Work out the finished part from the listing and answer in its coordinate system (mm). Coordinates: 2 decimals unless noted, no trailing zeros. Order: outer loops, then holes, each group sorted by start corner. A loop starts at its lowest first (then second) coordinate and runs counter-clockwise, first axis right, second up. Notation, with made-up numbers: (-31, 8) -> (-20, 8) arc R27 cw to (-20, 39) -> close; hole circle Ø3 at (-3, -37.5). An arc over 180 degrees is marked (long way). Use one line per item in the form item = value.
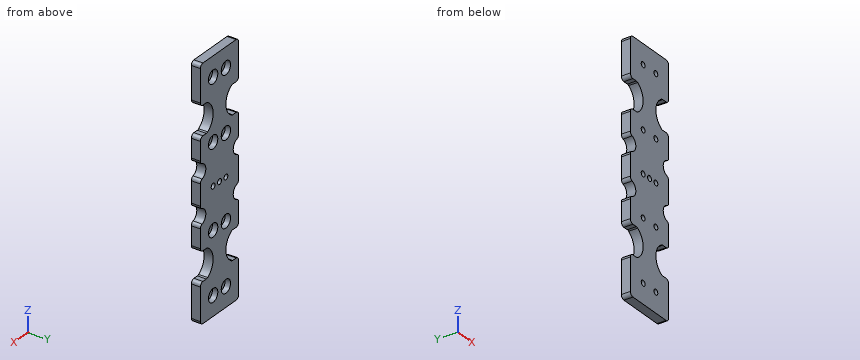
Autodesk Inventor part; units mm, degrees
ref_plane "YZ Plane" through (0, 0, 0) normal (1, 0, 0) x (0, 1, 0)
ref_plane "XZ Plane" through (0, 0, 0) normal (0, 1, 0) x (-1, 0, 0)
ref_plane "XY Plane" through (0, 0, 0) normal (0, 0, 1) x (1, 0, 0)
sketch "Sketch1" plane through (0, 0, 0) normal (0, 1, 0) x (-1, 0, 0)
  line L0 (13.7897, -1.2319) -> (-9.6368, -1.2319) construction
  line L1 (0.7897, 10.3965) -> (0.7897, -17.2319) construction
  line L2 (0.7897, -1.2319) -> (15.7897, -1.2319)
  line L3 (15.7897, -1.2319) -> (15.7897, -7.0606)
  line L4 (15.7897, -8.7319) -> (0.7897, -8.7319)
  line L5 (0.7897, -8.7319) -> (0.7897, -1.2319)
  line L6 (21.7897, -1.2319) -> (-22.2103, -1.2319) construction
  line L7 (0.7897, 17.7681) -> (0.7897, -29.2319) construction
  circle A0 centre (5.7897, -24.2319) radius 3.65
  circle A1 centre (5.7897, -24.2319) radius 5
  circle A2 centre (5.7897, -58.2319) radius 3.65
  circle A3 centre (5.7897, -58.2319) radius 5
  line L8 (0.7897, -17.2319) -> (15.7897, -17.2319)
  line L9 (15.7897, -18.9033) -> (15.7897, -29.2319)
  line L10 (13.7897, -31.2319) -> (11.138, -31.2319)
  line L11 (0.7897, -31.2319) -> (0.7897, -17.2319)
  line L12 (0.7897, -51.2319) -> (15.7897, -51.2319)
  line L13 (15.7897, -51.2319) -> (15.7897, -65.2319)
  line L14 (15.7897, -65.2319) -> (0.7897, -65.2319)
  line L15 (0.7897, -65.2319) -> (0.7897, -51.2319)
  arc A4 (14.4297, -8.9554) -> (14.4297, -17.0085) centre (15.7897, -12.9819) ccw
  line L16 (15.7897, -51.2319) -> (0.7897, -51.2319)
  line L17 (0.7897, -51.2319) -> (0.7897, -47.2319)
  line L18 (11.138, -47.2319) -> (13.7897, -47.2319)
  line L19 (15.7897, -49.2319) -> (15.7897, -51.2319)
  line L20 (15.7897, -65.2319) -> (0.7897, -65.2319)
  line L21 (0.7897, -65.2319) -> (0.7897, -69.2319)
  line L22 (0.7897, -69.2319) -> (13.7897, -69.2319)
  line L23 (15.7897, -67.2319) -> (15.7897, -65.2319)
  arc A5 (14.4297, -8.9554) -> (15.7897, -7.0606) centre (13.7897, -7.0606) ccw
  arc A6 (15.7897, -18.9033) -> (14.4297, -17.0085) centre (13.7897, -18.9033) ccw
  arc A7 (-12.8503, -17.0085) -> (-14.2103, -18.9033) centre (-12.2103, -18.9033) ccw
  circle A8 centre (-4.2103, -24.2319) radius 3.65
  circle A9 centre (-4.2103, -24.2319) radius 5
  line L24 (0.7897, -17.2319) -> (-14.2103, -17.2319)
  arc A10 (-12.8503, -17.0085) -> (-12.8503, -8.9554) centre (-14.2103, -12.9819) ccw
  arc A11 (-14.2103, -7.0606) -> (-12.8503, -8.9554) centre (-12.2103, -7.0606) ccw
  line L25 (-14.2103, -8.7319) -> (0.7897, -8.7319)
  line L26 (-14.2103, -1.2319) -> (-14.2103, -7.0606)
  line L27 (-14.2103, -18.9033) -> (-14.2103, -29.2319)
  line L28 (-12.2103, -31.2319) -> (-9.5586, -31.2319)
  line L29 (-14.2103, -49.2319) -> (-14.2103, -51.2319)
  line L30 (-9.5586, -47.2319) -> (-12.2103, -47.2319)
  line L31 (0.7897, -51.2319) -> (-14.2103, -51.2319)
  line L32 (-14.2103, -51.2319) -> (0.7897, -51.2319)
  line L33 (-14.2103, -51.2319) -> (-14.2103, -65.2319)
  circle A12 centre (-4.2103, -58.2319) radius 3.65
  circle A13 centre (-4.2103, -58.2319) radius 5
  line L34 (-14.2103, -67.2319) -> (-14.2103, -65.2319)
  line L35 (-14.2103, -65.2319) -> (0.7897, -65.2319)
  line L36 (-14.2103, -65.2319) -> (0.7897, -65.2319)
  line L37 (0.7897, -69.2319) -> (-12.2103, -69.2319)
  line L38 (0.7897, 6.2681) -> (0.7897, -1.2319)
  arc A14 (-12.8503, 6.4915) -> (-12.8503, 14.5446) centre (-14.2103, 10.5181) ccw
  line L39 (-14.2103, 6.2681) -> (0.7897, 6.2681)
  line L40 (-14.2103, -1.2319) -> (-14.2103, 4.5967)
  arc A15 (-12.8503, 6.4915) -> (-14.2103, 4.5967) centre (-12.2103, 4.5967) ccw
  line L41 (15.7897, -1.2319) -> (15.7897, 4.5967)
  line L42 (15.7897, 6.2681) -> (0.7897, 6.2681)
  line L43 (0.7897, -12.8604) -> (0.7897, 14.7681) construction
  line L44 (0.7897, -20.2319) -> (0.7897, 26.7681) construction
  circle A16 centre (5.7897, 55.7681) radius 3.65
  circle A17 centre (5.7897, 55.7681) radius 5
  line L45 (0.7897, 48.7681) -> (15.7897, 48.7681)
  line L46 (15.7897, 48.7681) -> (15.7897, 62.7681)
  line L47 (15.7897, 62.7681) -> (0.7897, 62.7681)
  line L48 (0.7897, 62.7681) -> (0.7897, 48.7681)
  line L49 (15.7897, 48.7681) -> (0.7897, 48.7681)
  line L50 (11.138, 44.7681) -> (13.7897, 44.7681)
  line L51 (15.7897, 45.7681) -> (15.7897, 48.7681)
  line L52 (15.7897, 62.7681) -> (0.7897, 62.7681)
  line L53 (0.7897, 66.7681) -> (13.7897, 66.7681)
  line L54 (15.7897, 64.7681) -> (15.7897, 62.7681)
  line L55 (0.7897, 62.7681) -> (0.7897, 66.7681)
  line L56 (13.7897, 28.7681) -> (11.138, 28.7681)
  circle A18 centre (5.7897, 21.7681) radius 3.65
  circle A19 centre (5.7897, 21.7681) radius 5
  line L57 (0.7897, 14.7681) -> (15.7897, 14.7681)
  line L58 (15.7897, 16.4394) -> (15.7897, 27.7681)
  arc A20 (14.4297, 14.5446) -> (14.4297, 6.4915) centre (15.7897, 10.5181) ccw
  arc A21 (15.7897, 4.5967) -> (14.4297, 6.4915) centre (13.7897, 4.5967) ccw
  arc A22 (14.4297, 14.5446) -> (15.7897, 16.4394) centre (13.7897, 16.4394) ccw
  line L59 (0.7897, 14.7681) -> (-14.2103, 14.7681)
  arc A23 (-14.2103, 16.4394) -> (-12.8503, 14.5446) centre (-12.2103, 16.4394) ccw
  circle A24 centre (-4.2103, 21.7681) radius 3.65
  line L60 (-14.2103, 16.4394) -> (-14.2103, 26.7681)
  line L61 (-12.2103, 28.7681) -> (-9.5586, 28.7681)
  line L62 (0.7897, 28.7681) -> (0.7897, 14.7681)
  circle A25 centre (-4.2103, 21.7681) radius 5
  line L63 (0.7897, 66.7681) -> (-12.2103, 66.7681)
  line L64 (-14.2103, 64.7681) -> (-14.2103, 62.7681)
  line L65 (0.7897, 48.7681) -> (0.7897, 44.7681)
  circle A26 centre (-4.2103, 55.7681) radius 3.65
  line L66 (-14.2103, 62.7681) -> (0.7897, 62.7681)
  line L67 (-14.2103, 62.7681) -> (0.7897, 62.7681)
  line L68 (-14.2103, 48.7681) -> (-14.2103, 62.7681)
  line L69 (0.7897, 48.7681) -> (-14.2103, 48.7681)
  line L70 (-14.2103, 48.7681) -> (0.7897, 48.7681)
  line L71 (-14.2103, 46.7681) -> (-14.2103, 48.7681)
  line L72 (-9.5586, 44.7681) -> (-12.2103, 44.7681)
  circle A27 centre (-4.2103, 55.7681) radius 5
  arc A28 (15.7897, 64.7681) -> (13.7897, 66.7681) centre (13.7897, 64.7681) ccw
  arc A29 (-12.2103, 66.7681) -> (-14.2103, 64.7681) centre (-12.2103, 64.7681) ccw
  arc A30 (13.7897, -69.2319) -> (15.7897, -67.2319) centre (13.7897, -67.2319) ccw
  arc A31 (-14.2103, -67.2319) -> (-12.2103, -69.2319) centre (-12.2103, -67.2319) ccw
  arc A32 (10.0879, 44.4702) -> (10.0879, 29.0659) centre (14.8397, 36.7681) ccw
  line L73 (15.7897, 46.7681) -> (15.7897, 45.7681)
  line L74 (15.7897, 26.7681) -> (15.7897, 27.7681)
  arc A33 (13.7897, 44.7681) -> (15.7897, 46.7681) centre (13.7897, 46.7681) ccw
  arc A34 (11.138, 44.7681) -> (10.0879, 44.4702) centre (11.138, 42.7681) ccw
  arc A35 (10.0879, 29.0659) -> (11.138, 28.7681) centre (11.138, 30.7681) ccw
  arc A36 (15.7897, 26.7681) -> (13.7897, 28.7681) centre (13.7897, 26.7681) ccw
  arc A37 (-8.5085, 29.0659) -> (-8.5085, 44.4702) centre (-13.2603, 36.7681) ccw
  line L75 (-14.2103, 45.7681) -> (-14.2103, 44.7681)
  line L76 (-14.2103, 27.7681) -> (-14.2103, 28.7681)
  arc A38 (-8.5085, 44.4702) -> (-9.5586, 44.7681) centre (-9.5586, 42.7681) ccw
  arc A39 (-9.5586, 28.7681) -> (-8.5085, 29.0659) centre (-9.5586, 30.7681) ccw
  arc A40 (-12.2103, 28.7681) -> (-14.2103, 26.7681) centre (-12.2103, 26.7681) ccw
  arc A41 (-14.2103, 46.7681) -> (-12.2103, 44.7681) centre (-12.2103, 46.7681) ccw
  arc A42 (10.0879, -31.5298) -> (10.0879, -46.9341) centre (14.8397, -39.2319) ccw
  arc A43 (-8.5085, -46.9341) -> (-8.5085, -31.5298) centre (-13.2603, -39.2319) ccw
  line L77 (-14.2103, -30.2319) -> (-14.2103, -31.2319)
  line L78 (-14.2103, -47.2319) -> (-14.2103, -48.2319)
  line L79 (15.7897, -30.2319) -> (15.7897, -31.2319)
  line L80 (15.7897, -47.2319) -> (15.7897, -48.2319)
  arc A44 (13.7897, -31.2319) -> (15.7897, -29.2319) centre (13.7897, -29.2319) ccw
  arc A45 (15.7897, -49.2319) -> (13.7897, -47.2319) centre (13.7897, -49.2319) ccw
  arc A46 (10.0879, -46.9341) -> (11.138, -47.2319) centre (11.138, -45.2319) ccw
  arc A47 (11.138, -31.2319) -> (10.0879, -31.5298) centre (11.138, -33.2319) ccw
  arc A48 (-9.5586, -47.2319) -> (-8.5085, -46.9341) centre (-9.5586, -45.2319) ccw
  arc A49 (-12.2103, -47.2319) -> (-14.2103, -49.2319) centre (-12.2103, -49.2319) ccw
  arc A50 (-8.5085, -31.5298) -> (-9.5586, -31.2319) centre (-9.5586, -33.2319) ccw
  arc A51 (-14.2103, -29.2319) -> (-12.2103, -31.2319) centre (-12.2103, -29.2319) ccw
  circle A52 centre (5.7897, 55.7681) radius 1.5
  circle A53 centre (-4.2103, 55.7681) radius 1.5
  circle A54 centre (5.7897, 21.7681) radius 1.5
  circle A55 centre (-4.2103, 21.7681) radius 1.5
  circle A56 centre (5.7897, -24.2319) radius 1.5
  circle A57 centre (-4.2103, -24.2319) radius 1.5
  circle A58 centre (5.7897, -58.2319) radius 1.5
  circle A59 centre (-4.2103, -58.2319) radius 1.5
  circle A60 centre (0.7897, -1.2319) radius 1.5
  circle A61 centre (5.7897, -1.2319) radius 1.5
  circle A62 centre (-4.2103, -1.2319) radius 1.5
  point P0 (0, 0)
  point P1 (15.7897, -69.2319)
  point P2 (-14.2103, -69.2319)
  point P3 (15.7897, 44.7681)
  point P4 (15.7897, 66.7681)
  point P5 (15.7897, 28.7681)
  point P6 (-14.2103, 66.7681)
  point P7 (10.6085, 44.7681)
  point P8 (10.6085, 28.7681)
  point P9 (-9.0292, 28.7681)
  point P10 (-9.0292, 44.7681)
  point P11 (10.6085, -31.2319)
  point P12 (10.6085, -47.2319)
  point P13 (-9.0292, -31.2319)
  point P14 (-9.0292, -47.2319)
  dimension "d0" = 15
  dimension "d1" = 7.5
  dimension "d2" = 7.3
  dimension "d3" = 23
  dimension "d4" = 10
  dimension "d5" = 7.3
  dimension "d6" = 10
  dimension "d7" = 34
  dimension "d8" = 4
  dimension "d9" = 4
  dimension "d10" = 2
  dimension "d11" = 2
  dimension "d12" = 2
  dimension "d13" = 2
  dimension "d14" = 2
  dimension "d19" = 3
  dimension "d20" = 3
  dimension "d21" = 3
  dimension "d22" = 3
  dimension "d23" = 3
  dimension "d24" = 3
  dimension "d25" = 3
  dimension "d26" = 3
  dimension "d27" = 3
  dimension "d28" = 3
  dimension "d29" = 3
extrude "Extrusion1" add sketch "Sketch1" along normal blind 5 contours A60 L38 L42 A21 L41 L2 A61 | L2 A61 L3 A5 L4 L5 A60 | L5 L25 A11 L26 L40 A15 L39 L38 A60 | L4 A5 A4 A6 L8 L24 A7 A10 A11 L25 | L39 A15 A14 A23 L59 L57 A22 A20 A21 L42 | A1 | A9 | A6 L9 A44 L10 A47 A42 A46 L18 A45 L19 L12 L31 L29 A49 L30 A48 A43 A50 L28 A51 L27 A7 L24 L8 | A25 | A19 | A23 L60 A40 L61 A39 A37 A38 L72 A41 L71 L69 L45 L51 A33 L50 A34 A32 A35 L56 A36 L58 A22 L57 L59 | A3 | L13 L14 L15 L12 | A13 | L31 L15 L35 L33 | A27 | L68 L66 L48 L69 | A17 | L45 L48 L47 L46 | L23 A30 L22 L21 L14 | L35 L21 L37 A31 L34 | L64 A29 L63 L55 L66 | L47 L55 L53 A28 L54
extrude "Extrusion2" add sketch "Sketch1" along normal blind 2 contours A0 | A2 | A8 | A12 | A16 | A18 | A24 | A26
properties part number "Stopper Lifter_3DPrint"
(1) Each of these flat-tipped pins is pushed along its axis until it touches: P1, Ø1.8, axis at x = 4.21, z = -58.23, coming from the +Y side; P2, Ø3.5, axis at x = -7, z = 56.5, coming from the +Y side. Where does it stop, or does it pass through?
Data:
P1 = through
P2 = 2
(2) Section B-B on z = 34.5 is taken. Write down the section's boundary in (x, y).
Data:
outline = (-6.08, 0) -> (4.5, 0) -> (4.5, 5) -> (-6.08, 5) -> close
(3) Section C-C on z = -45.5 is taken. Write down the section's boundary in (x, y), plus the area to 3 significant figures.
Data:
outline = (-8.31, 0) -> (6.73, 0) -> (6.73, 5) -> (-8.31, 5) -> close
area = 75.2 mm²
(4) Section A-A on y = 4.1 is taken. Count the separate pieces of the cut face and the enclosed holes in it, plus the area to 3 significant figures.
Data:
separate_pieces = 1
enclosed_holes = 11
area = 3,050 mm²
(5) Straight lines are drawn through the part: line 1 along X through (y, z) = (3.65, 55.5); line 2 along Z through (x, y) = (4, 2.9); line 3 along Z through (x, y) = (8.5, 2.2). For each, find the intervals that lie inside material, in ascending order.
Data:
line_1 = -15.79 to -9.43, -2.15 to 0.57, 7.85 to 14.21
line_2 = -69.23 to -61.88, -54.59 to -27.88, -20.59 to -2.72, 0.25 to 18.12, 25.41 to 52.12, 59.41 to 66.77
line_3 = -69.23 to -46.93, -31.54 to 29.07, 44.46 to 66.77
